Source: CAD feature listing. Evaluate the final solid. Frame: model axes, mm. A direction names the side the tool comes from. Round coordinates to 2 decimals unless told otherwise and drop trailing zeros. Order: outer loops, then holes, each group sorted by start corner. A loop starts at its lowest first (then second) coordinate and runs counter-clockwise, first axis right, second up. Notation, with made-up numbers: (60, 71.25) -> (67, 71.25) arc R22 ccw to (67, 79.25) -> close; hole circle Ø1 at (81.25, 54.5). An arc over 180 degrees is marked (long way). Answer as CSV lines item,"result". Start each with the question number.
(1) Section query C-C (z = -39). Output: boundary loops of the cut face in (x, y).
(2) Section query A-A (z = -22). Output: boundary loops of the cut face in (x, y).
(3) Section query B-B (x = 80). Output: boundary loops of the cut face in (y, z), plus the area to 3 significant figures.
(4) Line query: line 1 along X through (y, z) = (24, -38); line 2 along X through (y, z) = (8, -1.5); line 3 along Z through (x, y) = (5, 35.5). Output: solid intervals per line, ascending. Write a range as from..to.
(5) Contact query for flat-ended pins moving along their axis: P1, Ø17, axis at x = 21.66, y = 23.86, coming from the +Z side; P2, Ø3, axis at x = 74.5, y = 2, coming from the +Z side; P3, Ø7, axis at y = -16, z = -11.5, coming from the +X side. Output: stop coordinate, or through.
(6) Set-up query: faces 4 (the flat face through (4, 25.4, -20)), 5 (the flat face through (86, 0, -22)), 6 (the flat face through (47, 27, -0.745)), 7 (the flat face through (80, 27, -35.156)), 8 (the cylindrical face through (51.174, 38.348, -15.859)). Return all of +Z, -Z, +X, -X, +Y, -Y with unobstructed straight access to the full face (end or side cutting, diameter ignored); none if empty.
(7) Section query D-D (x = 40.5). Output: boundary loops of the cut face in (y, z).
(8) Pull-direction query (X, two-part tool) for faces 1 (the cylindrical face through (87.664, 21.375, -32.824)), 2 (the flat face through (69.85, -12, -4)), 3 (the flat face through (16, 0, -22)); classes: +X half, -X half, draft (parallel to the pull), parting line (faces both ways), or undercut.
```python
from build123d import *

# Parameters (mm, degrees)
JAW_SIDE_EXTRUDE_DEPTH                           = 101.6
SKETCH2_W                                        = 84.1248
SKETCH2_H                                        = 30.5562
HOLLOW_CUT_EXTRUDE_DEPTH                         = 37.592
SKETCH3_R                                        = 5.969
SCREW_BOSS_EXTRUDE_DEPTH                         = 29.811288
SKETCH5_W                                        = 38.1
SKETCH5_H                                        = 23.8252
FOOT_EXTRUDE_DEPTH                               = 82.804
CBORE_FOR_M6_PAN_HEAD_MACHINE_SCREW1_D           = 6.6
CBORE_FOR_M6_PAN_HEAD_MACHINE_SCREW1_CBORE_D     = 13
CBORE_FOR_M6_PAN_HEAD_MACHINE_SCREW1_CBORE_DEPTH = 4.6
SKETCH12_W                                       = 14.651439237
SKETCH12_H                                       = 5.842
TOP_TRIM_CUT_EXTRUDE3_DEPTH                      = 120.902057968
SKETCH13_W                                       = 23.442855491
SKETCH13_H                                       = 12.95199816
WEB_TRIM_1_CUT_EXTRUDE4_DEPTH                    = 8.7376
SKETCH14_W                                       = 37.878491239
SKETCH14_H                                       = 12.95199816
WEB_TRIM_2_CUT_EXTRUDE5_DEPTH                    = 8.7376


with BuildPart() as part:
    # Sketch1 → Jaw side extrude (new body)
    with BuildSketch(Plane(origin=(0, 0, 0), x_dir=(0, 0, -1), z_dir=(1, 0, 0))):
        with BuildLine():
            Line((35.433, 45.212), (35.433, 43.647675453))
            ThreePointArc((35.433, 43.647675453), (34.258233808, 40.336625769), (31.259334135, 38.5064))
            ThreePointArc((31.259334135, 38.5064), (8.79859819, 24.798633085), (0, 0))
            Line((0, 0), (44.831, 0))
            Line((44.831, 0), (44.831, 45.212))
            Line((44.831, 45.212), (35.433, 45.212))
        make_face()
    extrude(amount=JAW_SIDE_EXTRUDE_DEPTH)

    # Sketch2 → Hollow cut extrude (cut)
    with BuildSketch(Plane(origin=(0, 45.212, 0), x_dir=(1, 0, 0), z_dir=(0, 1, 0))):
        with Locations((50.8, 15.2781)):
            Rectangle(SKETCH2_W, SKETCH2_H)
    extrude(amount=-HOLLOW_CUT_EXTRUDE_DEPTH, mode=Mode.SUBTRACT)

    # Sketch3 → Screw boss extrude (add)
    with BuildSketch(Plane.XY.offset(-30.5562)):
        with BuildLine():
            Line((67.818, 7.62), (67.818, 21.33399816))
            ThreePointArc((67.818, 21.33399816), (50.8, 38.35199816), (33.782, 21.33399816))
            Line((33.782, 21.33399816), (33.782, 7.62))
            Line((33.782, 7.62), (67.818, 7.62))
        make_face()
        with Locations((50.8, 21.33399816)):
            Circle(SKETCH3_R, mode=Mode.SUBTRACT)
    extrude(amount=SCREW_BOSS_EXTRUDE_DEPTH)

    # Sketch5 → Foot extrude (add)
    with BuildSketch(Plane(origin=(0, 0, -44.831), x_dir=(-1, 0, 0), z_dir=(0, 0, -1))):
        with Locations((-50.8, -11.9126)):
            Rectangle(SKETCH5_W, SKETCH5_H)
    extrude(amount=-FOOT_EXTRUDE_DEPTH)

    # CBORE for M6 Pan Head Machine Screw1 (through all)
    with Locations(Plane(origin=(50.8, -38.1, -30.5562), x_dir=(1, 0, 0), z_dir=(0, 0, 1))):
        with Locations((-29.14300736, 61.964884424), (30.859893074, 61.964884424)):
            CounterBoreHole(CBORE_FOR_M6_PAN_HEAD_MACHINE_SCREW1_D / 2, CBORE_FOR_M6_PAN_HEAD_MACHINE_SCREW1_CBORE_D / 2, CBORE_FOR_M6_PAN_HEAD_MACHINE_SCREW1_CBORE_DEPTH)

    # Sketch12 → top trim Cut-Extrude3 (cut, through all)
    with BuildSketch(Plane.ZY):
        with Locations((-37.505280382, 42.291)):
            Rectangle(SKETCH12_W, SKETCH12_H)
    extrude(amount=-TOP_TRIM_CUT_EXTRUDE3_DEPTH, mode=Mode.SUBTRACT)

    # Sketch13 → web trim 1 Cut-Extrude4 (cut)
    with BuildSketch(Plane.ZY.offset(-8.7376)):
        with Locations((-18.834772254, 31.87599908)):
            Rectangle(SKETCH13_W, SKETCH13_H)
    extrude(amount=WEB_TRIM_1_CUT_EXTRUDE4_DEPTH, mode=Mode.SUBTRACT)

    # Sketch14 → web trim 2 Cut-Extrude5 (cut)
    with BuildSketch(Plane(origin=(92.8624, 0, 0), x_dir=(0, 0, -1), z_dir=(1, 0, 0))):
        with Locations((11.616954381, 31.87599908)):
            Rectangle(SKETCH14_W, SKETCH14_H)
    extrude(amount=WEB_TRIM_2_CUT_EXTRUDE5_DEPTH, mode=Mode.SUBTRACT)


solid = part.part
```
Answer block:
1,outline,"(0, 0) -> (31.75, 0) -> (31.75, -23.83) -> (69.85, -23.83) -> (69.85, 0) -> (101.6, 0) -> (101.6, 39.37) -> (0, 39.37) -> close; hole circle Ø6.6 at (21.66, 23.86); hole circle Ø6.6 at (81.66, 23.86)"
2,outline,"(0, 0) -> (31.75, 0) -> (31.75, -23.83) -> (69.85, -23.83) -> (69.85, 0) -> (101.6, 0) -> (101.6, 25.4) -> (92.86, 25.4) -> (92.86, 7.62) -> (67.82, 7.62) -> (67.82, 21.33) arc R17.02 ccw to (33.78, 21.33) -> (33.78, 7.62) -> (8.74, 7.62) -> (8.74, 25.4) -> (0, 25.4) -> close; hole circle Ø11.94 at (50.8, 21.33)"
3,outline,"(0, -44.83) -> (21.01, -44.83) -> (21.01, -35.16) -> (17.58, -35.16) -> (17.58, -30.56) -> (7.62, -30.56) -> (7.62, -0.74) arc R39.35 ccw to (0, 0) -> close; (26.72, -44.83) -> (39.37, -44.83) -> (39.37, -33.23) arc R5.25 cw to (38.51, -31.26) arc R39.35 ccw to (38.35, -30.56) -> (30.15, -30.56) -> (30.15, -35.16) -> (26.72, -35.16) -> close"
3,area,"678 mm2"
4,line 1,"0..18.36, 24.95..78.36, 84.96..101.6"
4,line 2,"0..8.74, 33.78..67.82, 92.86..101.6"
4,line 3,"-44.83..-30.56"
5,P1,"z = -30.56"
5,P2,"z = 0"
5,P3,"x = 69.85"
6,face 4,"+Z, -X, +Y"
6,face 5,"+Z, -Z, +X, -Y"
6,face 6,"+Z, +X, -X, +Y"
6,face 7,"+Z"
6,face 8,"+Z, +Y"
7,outline,"(-23.83, -44.83) -> (39.37, -44.83) -> (39.37, -33.23) arc R5.25 cw to (38.51, -31.26) arc R39.35 ccw to (38.35, -30.56) -> (34.88, -30.56) -> (34.88, -0.74) -> (7.62, -0.74) arc R39.35 ccw to (0, 0) -> (0, 37.97) -> (-23.83, 37.97) -> close"
8,face 1,"undercut"
8,face 2,"+X half"
8,face 3,"draft"
